Autodesk Inventor part; units mm, degrees
ref_plane "Work Plane1" through (-7, 0, 0) normal (1, 0, 0) x (0, 1, 0)
ref_plane "XZ Plane" through (0, 0, 0) normal (0, 1, 0) x (-1, 0, 0)
ref_plane "XY Plane" through (0, 0, 0) normal (0, 0, 1) x (1, 0, 0)
sketch "Sketch1" plane through (0, 0, 0) normal (0, 0, 1) x (1, 0, 0)
  circle A0 centre (0, 0) radius 7
  dimension "d0" = 14
extrude "Extrusion1" add sketch "Sketch1" along normal blind 52
hole "Hole1" at (0, 0, 52) direction (0, 0, -1) diameter 3 depth 13
ref_plane "Work Plane1" through (-7, 0, 0) normal (1, 0, 0) x (0, 1, 0)
sketch "Sketch2" plane through (-7, 0, 0) normal (1, 0, 0) x (0, 1, 0)
  line L0 (-2.5, 29.5) -> (-2.5, 52)
  line L1 (-2.5, 52) -> (2.5, 52)
  line L2 (2.5, 52) -> (2.5, 29.5)
  line L3 (7, 52) -> (-7, 52)
  line L4 (7, 52) -> (-7, 52)
  line L5 (-7, 0) -> (7, 0)
  line L6 (7, 0) -> (7, 52)
  line L7 (-7, 0) -> (-7, 52)
  arc A0 (-2.5, 29.5) -> (2.5, 29.5) centre (0, 29.5) ccw
  point P0 (0, 0)
  point P1 (0, 27)
  dimension "d12" = 5
  dimension "d14" = 0
extrude "Extrusion2" cut sketch "Sketch2" along normal blind 3 contours L0 L1 L2 A0
chamfer "Chamfer1" distance 1 angle 45 2 edges at (1.2711, -6.8836, 52) (1.2711, 6.8836, 52)
properties part number "Shaft" material "Steel"
The listing builds one solid part. Answer for the finished solid, in the listing's coordinates (mm). A direction names the side the tool comes from. Give positions to 0.01 mm unless a question says otherwise; leave off trailing zeros. Order: outer loops, then holes, each group sorted by start corner. A loop starts at its lowest first (then second) coordinate and runs counter-clockwise, first axis right, second up. Notation, with made-up numbers: (12, 5.5) - (57, 5.5) arc R24 cw to (57, 43.5) - close; hole circle Ø6 at (35, -1). An arc over 180 degrees is marked (long way). Use one line per item in the form item = value. Start each with the question number.
(1) For faces 1 (the flat face through (1.5, -1.2, 52)), 2 (the flat face through (0, 0, 39)), 3 (the flat face through (-4, 0, 40)), determine the directions among +Z, -Z, +X, -X, +Y, -Y from which every point of the face is accessible in a straight line to the end or side of a thin tool.
(2) A cutting plane is placed at D-D, the plane z = 35. Write down the section's boundary in (x, y).
(3) A cutting plane is placed at C-C, the plane z = 44.5. Write down the section's boundary in (x, y).
(4) Consider line 1 (X direction, y = 0, z = 46.5); line 2 (Y direction, x = 0, z = 49.25); line 3 (Z direction, x = 1, y = 0.5). Determine where each line is inside the solid, lowest interval first. Write a range as from..to.
(5) The mould has two halves that part along X. Classify faces 4 (the flat face through (-5, -2.5, 41)), 5 (the cylindrical face through (-0.07, 1.5, 45.41)), 6 (the conical face through (6.169, 0.24, 51.826)): released by +X, released by -X, zero draft, split by the parting line, or undercut.
(6) A cutting plane is placed at B-B, the plane x = 0. Write down the section's boundary in (y, z).
(7) Flat-ended cylindrical pins translate along their axes: pin 1 Ø1.5 at (y, z) = (3.5, 13.5) entering from -X; pin 2 Ø0.8 at (x, z) = (-5.5, 43) entering from -Y; pin 3 Ø3 at (y, z) = (0.5, 29) entering from -X. Find the tip coordinate at first contact, or state that the pin passes through.
(8) A cutting plane is placed at A-A, the plane y = 0. Write down the section's boundary in (x, z).
Ans:
q1.face_1 = +Z, +X, -X, +Y, -Y
q1.face_2 = +Z
q1.face_3 = +Z, -X
q2.outline = (-6.54, -2.5) arc R7 ccw (long way) to (-6.54, 2.5) - (-4, 2.5) - (-4, -2.5) - close
q3.outline = (-6.54, -2.5) arc R7 ccw (long way) to (-6.54, 2.5) - (-4, 2.5) - (-4, -2.5) - close; hole circle Ø3 at (0, 0)
q4.line_1 = -4..-1.5, 1.5..7
q4.line_2 = -7..-1.5, 1.5..7
q4.line_3 = 0..39
q5.face_4 = zero draft
q5.face_5 = undercut
q5.face_6 = split by the parting line
q6.outline = (-7, 0) - (7, 0) - (7, 51) - (6, 52) - (1.5, 52) - (1.5, 39) - (-1.5, 39) - (-1.5, 52) - (-6, 52) - (-7, 51) - close
q7.pin_1 = -6.44
q7.pin_2 = -4.79
q7.pin_3 = -4
q8.outline = (-7, 0) - (7, 0) - (7, 51) - (6, 52) - (1.5, 52) - (1.5, 39) - (-1.5, 39) - (-1.5, 52) - (-4, 52) - (-4, 27) - (-7, 27) - close
